Can you work these out from the drawing? Everything is in mm from the part's minimum corner. A direction names the side the tool comes from. Coordinates: 2 decimals unless noted, no trailing zeros. Loops run counter-clockwise (first coordinate to the right, second up) from the corner with the lowest first, then second, coordinate; pieces in that order, holes last. Notation, with made-up numbers: (53.5, -22.75) - (86.5, -22.75) arc R21 cw to (86.5, -16.75) - close; hole circle Ø2 at (-22, -3.5). An arc over 180 degrees is marked (long way). Put each result on its own line as item: value. Start each with the question number.
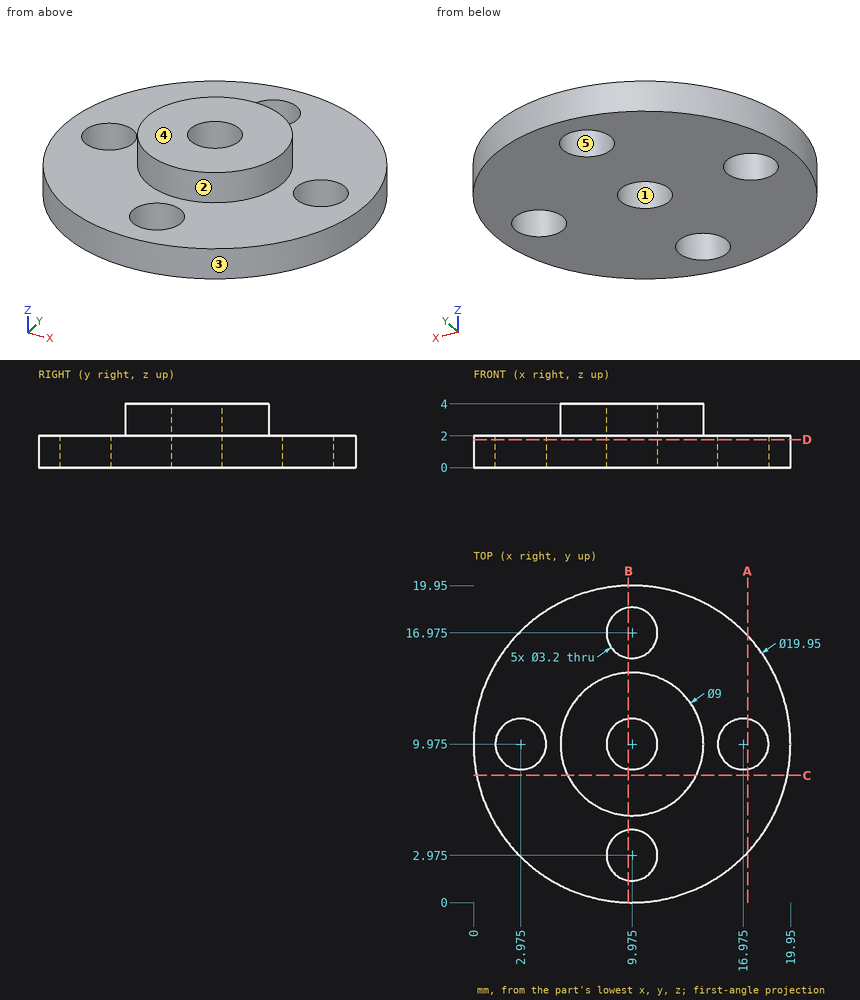
Q1. Please list where these lines run through material, in increasing order: line 1 along X through (y, z) = (10, 0.9); line 2 along X through (y, z) = (9.5, 1.4); line 3 along Y through (x, z) = (9.25, 0.9). Write a range as [from, to].
Q2. I want a section at D-D on z = 1.75. List the corners of the cut face in (x, y) for me (3 decimals), and give its area (3 significant figures).
Q3. On a 3-axis mill with a long thin cutter (end or side, diameter ignored), from which of +Z, -Z, +X, -X, +Y, -Y can I reach the whole of each face in a straight line? I mean the marked faces 1 and 2. Say none if no direction works.
Q4. I want a section at B-B on x = 9.75. List the corners of the cut face in (y, z) for me, and give its area (3 significant figures).
Q5. I want a section at C-C on y = 8. List the corners of the cut face in (x, z) for me.
Q6. We'd pull the mould along X, two halves only. Please class the marked faces 3, 4 and 5: released by +X, released by -X, zero draft, split by the parting line, or undercut.
Q7. Will these pins go through, and if not, where does the flat tip stop? pin 1 (2 mm diameter, centred on y = 15.5, z = 1, fed in from +X); pin 2 (1 mm diameter, centred on x = 7.5, z = 1.5, fed in from +Y); pin 3 (1 mm diameter, centred on x = 17.5, z = 2, fed in from +Y).
Q8. I want a section at A-A on x = 17.25. List the corners of the cut face in (y, z) for me.
Calculated:
1. line 1: [0, 1.38], [4.57, 8.38], [11.57, 15.38], [18.57, 19.95]
1. line 2: [0.01, 1.45], [4.5, 8.45], [11.5, 15.45], [18.5, 19.94]
1. line 3: [0.03, 1.55], [4.4, 8.55], [11.4, 15.55], [18.4, 19.92]
2. outline: circle Ø19.95 at (9.975, 9.975); hole circle Ø3.2 at (2.975, 9.975); hole circle Ø3.2 at (9.975, 2.975); hole circle Ø3.2 at (9.975, 9.975); hole circle Ø3.2 at (9.975, 16.975); hole circle Ø3.2 at (16.975, 9.975)
2. area: 272 mm2
3. face 1: +Z, -Z
3. face 2: +Z
4. outline: (0, 0) - (1.39, 0) - (1.39, 2) - (0, 2) - close; (4.56, 0) - (8.39, 0) - (8.39, 4) - (5.48, 4) - (5.48, 2) - (4.56, 2) - close; (11.56, 0) - (15.39, 0) - (15.39, 2) - (14.47, 2) - (14.47, 4) - (11.56, 4) - close; (18.56, 0) - (19.95, 0) - (19.95, 2) - (18.56, 2) - close
4. area: 32.5 mm2
5. outline: (0.2, 0) - (19.75, 0) - (19.75, 2) - (14.02, 2) - (14.02, 4) - (5.93, 4) - (5.93, 2) - (0.2, 2) - close
6. face 3: split by the parting line
6. face 4: zero draft
6. face 5: undercut
7. pin 1: x = 18.86
7. pin 2: y = 19.75
7. pin 3: y = 17.06
8. outline: (3.15, 0) - (8.4, 0) - (8.4, 2) - (3.15, 2) - close; (11.55, 0) - (16.8, 0) - (16.8, 2) - (11.55, 2) - close
